Autodesk Inventor part; units mm, degrees
ref_plane "YZ Plane" through (0, 0, 0) normal (1, 0, 0) x (0, 1, 0)
ref_plane "XZ Plane" through (0, 0, 0) normal (0, 1, 0) x (-1, 0, 0)
ref_plane "XY Plane" through (0, 0, 0) normal (0, 0, 1) x (1, 0, 0)
sketch "Boceto1" plane through (0, 0, 0) normal (0, 1, 0) x (-1, 0, 0)
  line L0 (50, -16) -> (50, -16.5)
  line L1 (50, -16.5) -> (49.0807, -16.5)
  circle A0 centre (0, -33) radius 1.5
  circle A1 centre (0, -33) radius 3
  arc A2 (0, -26) -> (5.7446, -37) centre (0, -33) ccw
  line L2 (5.7446, -37) -> (35, -37)
  line L3 (35, -37) -> (50, -19)
  line L4 (0, -23) -> (20, -23)
  line L5 (20, -23) -> (20, -17)
  line L6 (20, -17) -> (50, -17)
  line L7 (50, -17) -> (50, -19)
  line L8 (0, -31.5) -> (0, -30)
  line L9 (0, -26) -> (0, -23)
  point P0 (0, -37)
  dimension "d9" = 0.5
extrude "Extrusión1" add sketch "Boceto1" along normal blind 8 contours A1 | L9 L4 L5 L6 L7 L3 L2 A2
sketch "Boceto6" plane through (0, 0, 0) normal (0, -1, 0) x (1, 0, 0)
  line L0 (-50, -17) -> (-20, -17)
  line L1 (-50, -16) -> (-50, -14)
  line L2 (-50, -17) -> (-50, -16)
  line L3 (-50, -16.5) -> (-16.403, -16.5)
  line L4 (-20, -23) -> (-25, -23)
  line L5 (-5.7446, -37) -> (-35, -37)
  line L6 (-25, -23) -> (-25, -28)
  line L7 (-25, -37) -> (-25, -32)
  line L8 (-25, -32) -> (-5.7446, -32)
  line L9 (-5.7446, -32) -> (-5.7446, -27.061)
  line L10 (-25, -28) -> (-5.7446, -28)
  line L11 (-35, -37) -> (-30, -37)
  line L12 (-30, -37) -> (-30, -32)
  line L13 (-30, -32) -> (-25, -32)
  line L14 (-50, -19) -> (-50, -17)
  line L15 (-50, -19) -> (-45, -19)
  line L16 (-30, -37) -> (-45, -19)
  line L17 (-45, -19) -> (-40, -19)
  line L18 (-30, -32) -> (-40.8333, -19)
  line L19 (-40.8333, -19) -> (-25, -19)
  line L20 (-25, -19) -> (-25, -28)
  line L21 (-30, -32) -> (-34.1667, -32)
  line L22 (-40.8333, -19) -> (-35.8333, -19)
  line L23 (-35.8333, -19) -> (-25, -32)
  line L24 (-35.8333, -19) -> (-30.8333, -19)
  line L25 (-25, -32) -> (-20, -32)
  line L26 (-20, -32) -> (-30.8333, -19)
  line L27 (-30, 4) -> (-45, -14)
  line L28 (-45, -14) -> (-40, -14)
  line L29 (-30, -1) -> (-40.8333, -14)
  line L30 (-30, -1) -> (-34.1667, -1)
  line L31 (-35.8333, -14) -> (-25, -1)
  line L32 (-35.8333, -14) -> (-30.8333, -14)
  line L33 (-25, -1) -> (-20, -1)
  line L34 (-20, -1) -> (-30.8333, -14)
  point P0 (0, 0)
  dimension "d28" = 5
  dimension "d29" = 5
  dimension "d30" = 5
  dimension "d31" = 5
  dimension "d32" = 5
  dimension "d33" = 5
  dimension "d34" = 5
  dimension "d35" = 5
  dimension "d36" = 5
extrude "Extrusión6" cut sketch "Boceto6" against normal blind 10 contours L23 L19 L26 L6 L10 L8 | L21 L16 L17 L18 | L10 L6 L26 | L30 L29 L28 L27 | L31 L33 L34 L32
chamfer "Chaflán1" distance 2 angle 45 2 edges at (-50, 4, -19) (0, 4, -23)
sketch "Boceto9" plane through (0, 8, 0) normal (0, 1, 0) x (1, 0, 0)
  circle A0 centre (0, 33) radius 1.5
  circle A1 centre (0, 33) radius 2.6
  line L0 (0, 33) -> (0, 30.1)
  line L1 (0, 30.4) -> (0, 30.4753)
  line L2 (0, 30.4753) -> (0.263, 30.4753)
  line L3 (0.263, 30.4753) -> (-0.263, 30.4753)
  line L4 (-0.263, 30.4753) -> (-0.263, 29.9607)
  line L5 (0.263, 30.4753) -> (0.263, 30.0075)
  line L6 (0, 30.4) -> (0, 30.1)
  line L7 (0, 30.1) -> (0.263, 30.4133)
  line L8 (0, 30.1) -> (-0.263, 30.4133)
  line L9 (0.694, 30.1843) -> (0.8744, 30.5514)
  line L10 (0.694, 30.1843) -> (0.3637, 30.4256)
  line L11 (1.3477, 30.4322) -> (1.435, 30.8318)
  line L12 (1.3477, 30.4322) -> (0.9692, 30.5874)
  line L13 (1.9231, 30.8293) -> (1.9121, 31.2383)
  line L14 (1.9231, 30.8293) -> (1.5184, 30.8895)
  line L15 (2.3867, 31.3526) -> (2.2782, 31.7471)
  line L16 (2.3867, 31.3526) -> (1.9794, 31.3142)
  line L17 (2.7115, 31.9716) -> (2.5118, 32.3287)
  line L18 (2.7115, 31.9716) -> (2.3253, 31.8368)
  line L19 (2.8789, 32.6504) -> (2.5995, 32.9493)
  line L20 (2.8789, 32.6504) -> (2.5361, 32.4271)
  line L21 (2.8789, 33.3496) -> (2.5361, 33.5729)
  line L22 (2.8789, 33.3496) -> (2.5995, 33.0507)
  line L23 (2.7115, 34.0284) -> (2.3253, 34.1632)
  line L24 (2.7115, 34.0284) -> (2.5118, 33.6713)
  line L25 (2.3867, 34.6474) -> (1.9794, 34.6858)
  line L26 (2.3867, 34.6474) -> (2.2782, 34.2529)
  line L27 (1.9231, 35.1707) -> (1.5184, 35.1105)
  line L28 (1.9231, 35.1707) -> (1.9121, 34.7617)
  line L29 (1.3477, 35.5678) -> (0.9692, 35.4126)
  line L30 (1.3477, 35.5678) -> (1.435, 35.1682)
  line L31 (0.694, 35.8157) -> (0.3637, 35.5744)
  line L32 (0.694, 35.8157) -> (0.8744, 35.4486)
  line L33 (0, 35.9) -> (-0.263, 35.5867)
  line L34 (0, 35.9) -> (0.263, 35.5867)
  line L35 (-0.694, 35.8157) -> (-0.8744, 35.4486)
  line L36 (-0.694, 35.8157) -> (-0.3637, 35.5744)
  line L37 (-1.3477, 35.5678) -> (-1.435, 35.1682)
  line L38 (-1.3477, 35.5678) -> (-0.9692, 35.4126)
  line L39 (-1.9231, 35.1707) -> (-1.9121, 34.7617)
  line L40 (-1.9231, 35.1707) -> (-1.5184, 35.1105)
  line L41 (-2.3867, 34.6474) -> (-2.2782, 34.2529)
  line L42 (-2.3867, 34.6474) -> (-1.9794, 34.6858)
  line L43 (-2.7115, 34.0284) -> (-2.5118, 33.6713)
  line L44 (-2.7115, 34.0284) -> (-2.3253, 34.1632)
  line L45 (-2.8789, 33.3496) -> (-2.5995, 33.0507)
  line L46 (-2.8789, 33.3496) -> (-2.5361, 33.5729)
  line L47 (-2.8789, 32.6504) -> (-2.5361, 32.4271)
  line L48 (-2.8789, 32.6504) -> (-2.5995, 32.9493)
  line L49 (-2.7115, 31.9716) -> (-2.3253, 31.8368)
  line L50 (-2.7115, 31.9716) -> (-2.5118, 32.3287)
  line L51 (-2.3867, 31.3526) -> (-1.9794, 31.3142)
  line L52 (-2.3867, 31.3526) -> (-2.2782, 31.7471)
  line L53 (-1.9231, 30.8293) -> (-1.5184, 30.8895)
  line L54 (-1.9231, 30.8293) -> (-1.9121, 31.2383)
  line L55 (-1.3477, 30.4322) -> (-0.9692, 30.5874)
  line L56 (-1.3477, 30.4322) -> (-1.435, 30.8318)
  line L57 (-0.694, 30.1843) -> (-0.3637, 30.4256)
  line L58 (-0.694, 30.1843) -> (-0.8744, 30.5514)
  point P0 (0, 0)
  dimension "d47" = 5.2
  dimension "d48" = 2.9
  dimension "d49" = 0.263
  dimension "d50" = 0.526
  dimension "d51" = 0.3
  dimension "d54" = 360
extrude "Extrusión9" cut sketch "Boceto9" against normal blind 2.9
properties part number "pinza  individuial sg996r con rosca"
Verification items for the finished model (mm, model axes). A direction names the side the tool comes from. Round coordinates to 2 decimals unless told otherwise and drop trailing zeros. Order: outer loops, then holes, each group sorted by start corner. A loop starts at its lowest first (then second) coordinate and runs counter-clockwise, first axis right, second up. Notation, with made-up numbers: (-38, 4.5) -> (9, 4.5) arc R25 cw to (9, 17.5) -> close; hole circle Ø3 at (75.5, -24.75). An arc over 180 degrees is marked (long way). Put each result on its own line as item: value. Start each with the question number.
(1) Draft check along Z on faces 4 (the face through (-1, 4, -24)), 5 (the face through (-49.37, 3.94, -18.74)), 6 (the face through (1.2, 5.1, -31.8)), 7 (the face through (-21, 8, -28)). Enter one of: +Z half, -Z half, draft (parallel to the pull), parting line (faces both ways), or undercut.
(2) Tool access check on faces 1 (the face through (-11, 4, -23)), 2 (the face through (-43, 4, -19)), 3 (the face through (-20, 4, -37)). Record the directions out of +Z, -Z, +X, -X, +Y, -Y that give a thin tool (end or side, any length) a straight path to the whole face; none if there is none.
(3) Section check B-B (z = -28). Enter the section's corners in (x, y), then the cut area to 3 significant figures.
(4) Section check A-A (y = 3.75). State how many separate pieces and enclosed holes the cut face has, then the cut area to 3 significant figures.
(5) Section check D-D (z = -37.75). Enter the section's corners in (x, y), then the cut area to 3 significant figures.
(6) Depth check by flat-ended pin: pin 1 Ø4 at (x, y) = (-12.5, 2.5) entering from +Z; pin 2 Ø8 at (x, z) = (0.5, -22.5) entering from +Y; pin 3 Ø4.5 at (x, y) = (-44, 4.5) entering from -Z; pin 4 Ø1.8 at (x, z) = (0, -33) entering from -Y. Enter the tip coordinate at first touch or a pass-through.
(7) Section check C-C (x = -13.5). Enter the section's corners in (y, z), then the cut area to 3 significant figures.
(8) Material ranges on line 1 along X through (y, z) = (0.5, -24); line 2 along X through (y, z) = (2, -19.5); line 3 along Z through (x, y) = (-25, 3.75), recorded low to high.
Completed:
1. face 4: +Z half
1. face 5: -Z half
1. face 6: undercut
1. face 7: draft
2. face 1: +Z, +X, +Y, -Y
2. face 2: +Y, -Y
2. face 3: -Z, -X, +Y, -Y
3. outline: (-42.5, 0) -> (-37.5, 0) -> (-37.5, 8) -> (-42.5, 8) -> close; (-33.33, 0) -> (-28.33, 0) -> (-28.33, 8) -> (-33.33, 8) -> close; (-23.33, 0) -> (4.9, 0) -> (4.9, 8) -> (-23.33, 8) -> close
3. area: 306 mm2
4. separate pieces: 1
4. enclosed holes: 3
4. area: 705 mm2
5. outline: (-5.14, 0) -> (5.14, 0) -> (5.14, 8) -> (-5.14, 8) -> close
5. area: 82.3 mm2
6. pin 1: stops at z = -23
6. pin 2: stops at y = 8
6. pin 3: stops at z = -28.9
6. pin 4: passes through
7. outline: (0, -37) -> (8, -37) -> (8, -23) -> (0, -23) -> close
7. area: 112 mm2
8. line 1: x = -45.83 to -40.83, -36.67 to -31.67, -26.67 to -1
8. line 2: x = -49.1 to -44.58, -40.42 to -35.42, -30.42 to -20
8. line 3: z = -37 to -32, -26 to -17
